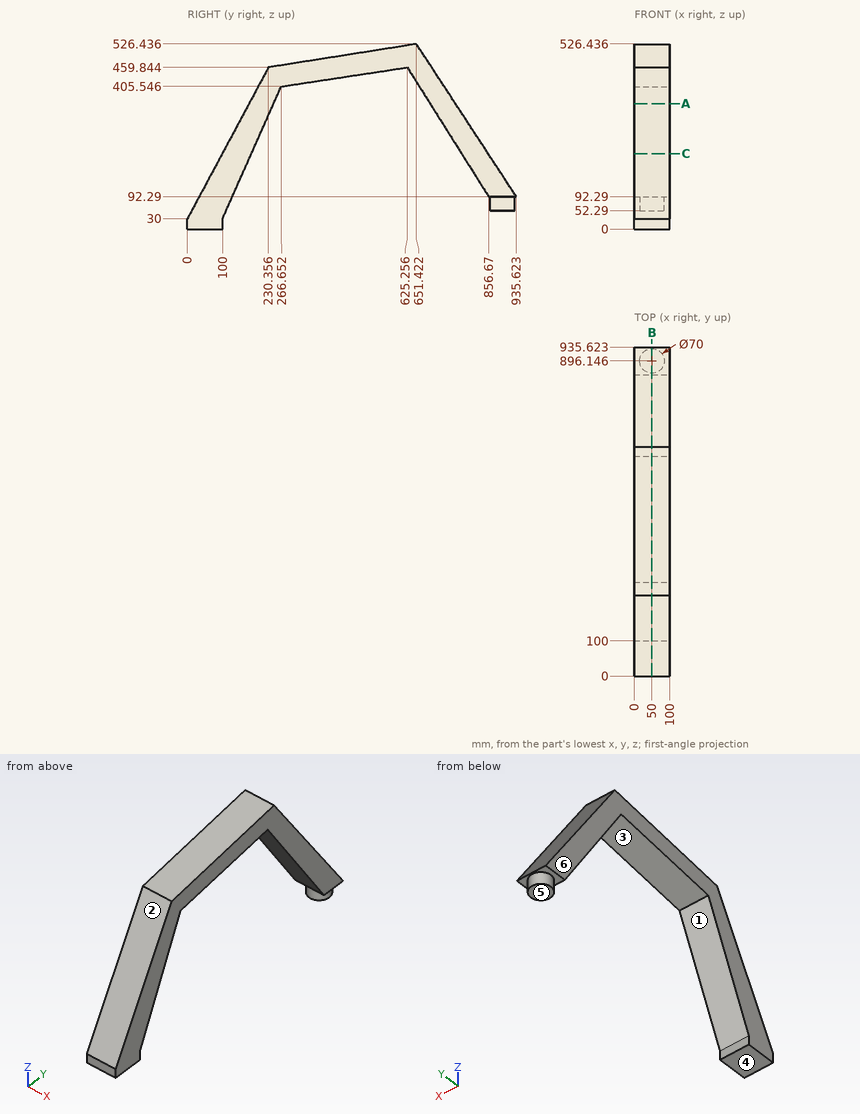
Part print with two shaded views. Sizes in mm from the minimum x, y, z corner. A direction names the side the tool comes from. Round coordinates to 2 decimals unless told otherwise and drop trailing zeros. Order: outer loops, then holes, each group sorted by start corner. A loop starts at its lowest first (then second) coordinate and runs counter-clockwise, first axis right, second up. Notation, with made-up numbers: (3.5, 43) - (45.5, 43) arc R30 ccw to (45.5, 74) - close; hole circle Ø1 at (-25.75, -14.5). An arc over 180 degrees is marked (long way). Answer in a Markdown table with one row per item. Add a question column.
(1) Band-saw the part on A-A on z = 357. List the corners of the cut face in (x, y), and give its area (3 significant figures).
(2) Band-saw the part on B-B on x = 50. List the corners of the cut face in (y, z) (1 decimal).
(3) Probe L1, parallel to Y at x = 26, z = 174 (1 decimal); L2, parallel to Y at x = 76, z = 351 (1 decimal); L3, parallel to Z at x = 11.5, y = 204.5 (1 decimal). List the from-to ranges inside material, lowest first. Write a range as [from, to].
(4) Mould opens along Y. For the marked faces 1, 2, 3 and 4 say: +Y half, -Y half, draft (parallel to the pull), parting line (faces both ways), or undercut.
(5) Drop flat-ended pins along their axis: pin 1 Ø8 at (x, z) = (88.5, 67) entering from -Y (1 decimal); pin 2 Ø1.5 at (x, y) = (39.5, 777.5) entering from -Z (1 decimal); pin 3 Ø8 at (x, z) = (63.5, 68) entering from +Y. Give the stop position or say it passes through.
(6) 3-axis set-ups, long thin cutter, end or side, ignore diameter. For the marked faces 5 and 6: which of +Z, -Z, +X, -X, +Y, -Y reach the whole face in a straight line?
(7) Band-saw the part on C-C on z = 214.5. List the corners of the cut face in (x, y) (1 decimal), and give its area (3 significant figures).
Data:
| question | item | result |
|---|---|---|
| 1 | outline | (0, 175.24) - (100, 175.24) - (100, 245.11) - (0, 245.11) - close; (0, 690.01) - (100, 690.01) - (100, 762.34) - (0, 762.34) - close |
| 1 | area | 14,200 mm^2 |
| 2 | outline | (0, 0) - (100, 0) - (100, 30) - (266.7, 405.5) - (625.3, 459.8) - (856.7, 92.3) - (861.1, 92.3) - (861.1, 52.3) - (931.1, 52.3) - (931.1, 92.3) - (935.6, 92.3) - (651.4, 526.4) - (230.4, 459.8) - (0, 30) - close |
| 3 | L1 | y = [77.2, 163.9], [805.2, 882.1] |
| 3 | L2 | y = [172, 242.4], [693.8, 766.3] |
| 3 | L3 | z = [265.5, 411.6] |
| 4 | face 1 | undercut |
| 4 | face 2 | -Y half |
| 4 | face 3 | undercut |
| 4 | face 4 | draft |
| 5 | pin 1 | stops at y = 17.7 |
| 5 | pin 2 | stops at z = 216.8 |
| 5 | pin 3 | stops at y = 929.83 |
| 6 | face 5 | -Z, +X, -X, +Y |
| 6 | face 6 | +Z, -Z, -X, +Y, -Y |
| 7 | outline | (0, 98.9) - (100, 98.9) - (100, 181.9) - (0, 181.9) - close; (0, 779.7) - (100, 779.7) - (100, 855.6) - (0, 855.6) - close |
| 7 | area | 15,900 mm^2 |
